Study the drawing (mm; zero at the part's minimum x, y, z) and answer. Round coordinates to 2 decimals unless told otherwise and drop trailing zeros. Write each loop counter-clockwise with the first axis right and the second up, starting at its lowest first coordinate (ties: lowest second). Pieces come first, ordered by that corner, then holes.
(1) Each of these flat-tipped pins is pushed along its axis until it touches: pin 1 Ø1.5 at (x, z) = (94.5, 2) entering from +Y; pin 2 Ø1.5 at (y, z) = (94, 1) entering from +X. Where does it stop, or does it pass through?
(2) A cutting plane is placed at C-C, the plane x = 24. Give the vertices of the cut face in (y, z).
(3) Find the intervals of material crossed by probe 1 along Y at (x, z) = (7.5, 2.35); probe 2 along X at (y, z) = (111, 1.75); probe 3 along X at (y, z) = (85, 2.35) (1 decimal), in increasing order.
(4) A cutting plane is placed at B-B, the plane z = 1.65. Give the number of separate pieces and of enclosed holes in the cut face.
(5) A cutting plane is placed at A-A, the plane y = 67. Give the vertices of the cut face in (x, z).
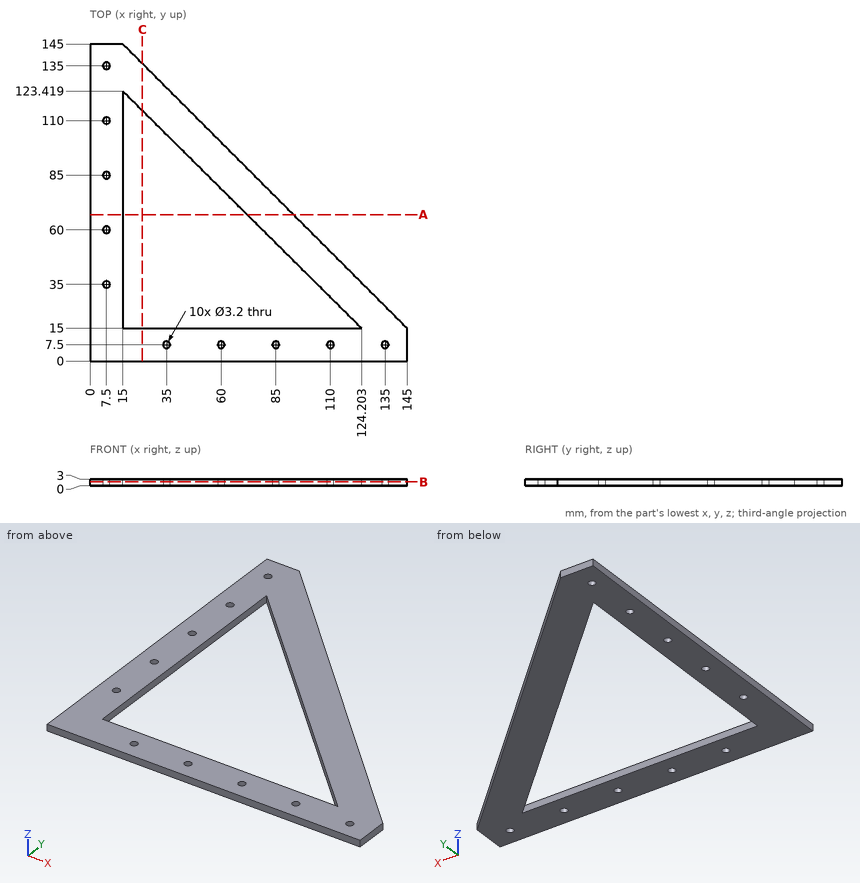
Solutions:
1. pin 1: stops at y = 66.25
1. pin 2: stops at x = 66.75
2. outline: (0, 0) - (15, 0) - (15, 3) - (0, 3) - close; (114.48, 0) - (136, 0) - (136, 3) - (114.48, 3) - close
3. probe 1: y = 0 to 33.4, 36.6 to 58.4, 61.6 to 83.4, 86.6 to 108.4, 111.6 to 133.4, 136.6 to 145
3. probe 2: x = 0 to 6.25, 8.75 to 15, 27.51 to 49
3. probe 3: x = 0 to 5.9, 9.1 to 15, 53.7 to 75
4. separate pieces: 1
4. enclosed holes: 11
5. outline: (0, 0) - (15, 0) - (15, 3) - (0, 3) - close; (71.83, 0) - (93, 0) - (93, 3) - (71.83, 3) - close
